CAD build for the part. Positions are in the model's coordinates, mm. A direction names the side the tool comes from. Coordinates: 2 decimals unless noted, no trailing zeros. Order: outer loops, then holes, each group sorted by start corner. A loop starts at its lowest first (then second) coordinate and runs counter-clockwise, first axis right, second up. Notation, with made-up numbers: (3.25, 30) -> (23.25, 30) arc R29 ccw to (23.25, 61) -> close; hole circle Ø11 at (45.5, 87.5). An arc over 180 degrees is marked (long way). Use one line per item in the form item = value. Start each with the question number.
from build123d import *

# Parameters (mm, degrees)
SKETCH1_R           = 6.35
BOSS_EXTRUDE1_DEPTH = 63.5
SKETCH2_R           = 3.175
CUT_EXTRUDE1_DEPTH  = 19.05
SKETCH5_W           = 1.1303
SKETCH5_H           = 6.35


with BuildPart() as part:
    # Sketch1 → Boss-Extrude1 (new body)
    with BuildSketch(Plane(origin=(0, 0, 0), x_dir=(1, 0, 0), z_dir=(0, 1, 0))):
        with Locations(Location((0, 0, 0), (0, 0, 270))):
            Circle(SKETCH1_R)
    extrude(amount=BOSS_EXTRUDE1_DEPTH)

    # Sketch2 → Cut-Extrude1 (cut)
    with BuildSketch(Plane(origin=(0, 0, 0), x_dir=(1, 0, 0), z_dir=(0, 1, 0))):
        with Locations(Location((0, 0, 0), (0, 0, 90))):
            Circle(SKETCH2_R)
    extrude(amount=CUT_EXTRUDE1_DEPTH, mode=Mode.SUBTRACT)

    # Sketch5 → #43 (0.089) Diameter Hole1 (revolve, cut)
    with BuildSketch(Plane(origin=(0, 9.525, 0), x_dir=(0, 1, 0), z_dir=(1, 0, 0))):
        with Locations((0.56515, 3.175)):
            Rectangle(SKETCH5_W, SKETCH5_H)
    revolve(axis=Axis((0, 9.525, -6.35), (0, 0, 1)), mode=Mode.SUBTRACT)


solid = part.part
1) 3-axis set-ups, long thin cutter, end or side, ignore diameter. For faces 1 (the face through (-0.95, 9.39, -3.03)), 2 (the face through (0, 63.5, 0)), 3 (the face through (0.43, 10.57, 4.68)): which of +Z, -Z, +X, -X, +Y, -Y reach the whole face in a straight line?
2) Cut at B-B on z = 0. Give the cut face in (x, y) (3 decimals), then the cut area to 3 significant figures.
3) Two-plate mould, pull along Z, no slides. Class faces 4 (the face through (-3.86, 31.31, -5.04)), 5 (the face through (3, 0, -2)), 6 (the face through (0, 19.05, 0)): released by +Z, released by -Z, zero draft, split by the parting line, or undercut.
4) Cut at A-A on x = 0. Give the cut face in (y, z) (3 decimals), then the cut area to 3 significant figures.
5) Probe L1, parallel to X at y = 10, z = 0 (3 decimals); L2, parallel to Y at x = 0, z = 4.2; L3, parallel to Y at x = 1.5, z = 1.25. List the from-to ranges inside material, lowest first.
6) Drop a flat-ended pin along its axis: P1, Ø3, axis at y = 54, z = 4.5, coming from the -X side. Give the stop position or say it passes through.
7) Cut at C-C on y = 36. Give the cut face in (x, z), then the cut area to 3 significant figures.
8) Cut at D-D on z = -2.5. Give the cut face in (x, y), then the cut area to 3 significant figures.
Values follow:
q1.face_1 = -Y
q1.face_2 = +Z, -Z, +X, -X, +Y
q1.face_3 = +Z
q2.outline = (-6.35, 0) -> (-3.175, 0) -> (-3.175, 19.05) -> (3.175, 19.05) -> (3.175, 0) -> (6.35, 0) -> (6.35, 63.5) -> (-6.35, 63.5) -> close
q2.area = 685 mm^2
q3.face_4 = split by the parting line
q3.face_5 = zero draft
q3.face_6 = undercut
q4.outline = (0, -6.35) -> (63.5, -6.35) -> (63.5, 6.35) -> (10.655, 6.35) -> (10.655, 3.175) -> (19.05, 3.175) -> (19.05, -3.175) -> (0, -3.175) -> close; (0, 3.175) -> (8.395, 3.175) -> (8.395, 6.35) -> (0, 6.35) -> close
q4.area = 678 mm^2
q5.L1 = -6.35 to -3.175, 3.175 to 6.35
q5.L2 = 0 to 8.39, 10.66 to 63.5
q5.L3 = 19.05 to 63.5
q6.P1 = -5.6
q7.outline = circle Ø12.7 at (0, 0)
q7.area = 127 mm^2
q8.outline = (-5.84, 0) -> (-1.96, 0) -> (-1.96, 19.05) -> (1.96, 19.05) -> (1.96, 0) -> (5.84, 0) -> (5.84, 63.5) -> (-5.84, 63.5) -> close
q8.area = 667 mm^2
